The listing builds one solid part. Answer for the finished solid, in the listing's coordinates (mm). A direction names the side the tool comes from. Coordinates: 2 decimals unless noted, no trailing zeros. Write each loop counter-clockwise with the first axis right and the second up, starting at its lowest first coordinate (ties: lowest second). Pieces come first, ordered by that corner, then holes.
from build123d import *

# Parameters (mm, degrees)
SKETCH1_W           = 22.6
SKETCH1_H           = 12.33
BOSS_EXTRUDE1_DEPTH = 16.09
SKETCH2_W           = 32.3
SKETCH2_H           = 12.33
BOSS_EXTRUDE2_DEPTH = 2.41
SKETCH3_W           = 22.6
SKETCH3_H           = 12.33
BOSS_EXTRUDE3_DEPTH = 4.23
BOSS_EXTRUDE4_DEPTH = 4.31
SKETCH5_R           = 3.335
BOSS_EXTRUDE5_DEPTH = 4.52
BOSS_EXTRUDE8_DEPTH = 2.18
SKETCH8_R           = 1.3
CUT_EXTRUDE3_DEPTH  = 4
SKETCH9_R           = 1.3
CUT_EXTRUDE4_DEPTH  = 4
SKETCH10_R          = 1
CUT_EXTRUDE5_DEPTH  = 10


with BuildPart() as part:
    # Sketch1 → Boss-Extrude1 (new body)
    with BuildSketch(Plane(origin=(0, 0, 0), x_dir=(1, 0, 0), z_dir=(0, 1, 0))):
        with Locations((11.3, 6.165)):
            Rectangle(SKETCH1_W, SKETCH1_H)
    extrude(amount=BOSS_EXTRUDE1_DEPTH)

    # Sketch2 → Boss-Extrude2 (add)
    with BuildSketch(Plane(origin=(0, 16.09, 0), x_dir=(1, 0, 0), z_dir=(0, 1, 0))):
        with Locations((11.25, 6.165)):
            Rectangle(SKETCH2_W, SKETCH2_H)
    extrude(amount=BOSS_EXTRUDE2_DEPTH)

    # Sketch3 → Boss-Extrude3 (add)
    with BuildSketch(Plane(origin=(0, 18.5, 0), x_dir=(1, 0, 0), z_dir=(0, 1, 0))):
        with Locations((11.3, 6.165)):
            Rectangle(SKETCH3_W, SKETCH3_H)
    extrude(amount=BOSS_EXTRUDE3_DEPTH)

    # Sketch4 → Boss-Extrude4 (add)
    with BuildSketch(Plane(origin=(0, 22.73, 0), x_dir=(1, 0, 0), z_dir=(0, 1, 0))):
        with BuildLine():
            ThreePointArc((0, 6.165), (6.165, 12.33), (12.33, 6.165))
            ThreePointArc((12.33, 6.165), (6.165, 0), (0, 6.165))
        make_face()
    extrude(amount=BOSS_EXTRUDE4_DEPTH)

    # Sketch5 → Boss-Extrude5 (add)
    with BuildSketch(Plane(origin=(0, 27.04, 0), x_dir=(1, 0, 0), z_dir=(0, 1, 0))):
        with Locations(Location((6.165, 6.165, 0), (0, 0, 270))):
            Circle(SKETCH5_R)
    extrude(amount=BOSS_EXTRUDE5_DEPTH)

    # Sketch6 → Boss-Extrude8 (add)
    with BuildSketch(Plane(origin=(0, 31.56, 0), x_dir=(1, 0, 0), z_dir=(0, 1, 0))):
        with BuildLine():
            ThreePointArc((9.455009686, 6.710949872), (6.165, 9.5), (2.874990314, 6.710949872))
            Line((2.874990314, 6.710949872), (2.83, 6.165))
            ThreePointArc((2.83, 6.165), (6.165, 2.83), (9.5, 6.165))
            Line((9.5, 6.165), (9.455009686, 6.710949872))
        make_face()
        with BuildLine():
            ThreePointArc((8.165, 22.365), (6.165, 24.365), (4.165, 22.365))
            Line((4.165, 22.365), (2.874990314, 6.710949872))
            ThreePointArc((2.874990314, 6.710949872), (6.165, 9.5), (9.455009686, 6.710949872))
            Line((9.455009686, 6.710949872), (8.165, 22.365))
        make_face()
    extrude(amount=BOSS_EXTRUDE8_DEPTH)

    # Sketch8 → Cut-Extrude3 (cut)
    with BuildSketch(Plane(origin=(0, 18.5, 0), x_dir=(1, 0, 0), z_dir=(0, 1, 0))):
        with Locations((-3.65, 6.165)):
            Circle(SKETCH8_R)
    extrude(amount=-CUT_EXTRUDE3_DEPTH, mode=Mode.SUBTRACT)

    # Sketch9 → Cut-Extrude4 (cut)
    with BuildSketch(Plane(origin=(0, 18.5, 0), x_dir=(1, 0, 0), z_dir=(0, 1, 0))):
        with Locations((26.15, 6.165)):
            Circle(SKETCH9_R)
    extrude(amount=-CUT_EXTRUDE4_DEPTH, mode=Mode.SUBTRACT)

    # Sketch10 → Cut-Extrude5 (cut)
    with BuildSketch(Plane(origin=(0, 33.74, 0), x_dir=(1, 0, 0), z_dir=(0, 1, 0))):
        with Locations(Location((6.165, 20.865, 0), (0, 0, 270))):
            Circle(SKETCH10_R)
    extrude(amount=-CUT_EXTRUDE5_DEPTH, mode=Mode.SUBTRACT)


solid = part.part
Q1. Which of the six approach directions +Z, -Z, +X, -X, +Y, -Y give full straight-line access (tool end or side, diameter ignored) to faces 1 (the face through (-2, 18.5, -6)), 2 (the face through (0, 8, -6)), 3 (the face through (11.86, 24.85, -8.53))?
Answers below:
face 1: +Z, -Z, -X, +Y
face 2: +Z, -Z, -X, -Y
face 3: none
Q2. Determine the mould class of faces 4 (the face through (27.4, 17, -9)), 5 (the face through (6.209, 32.635, -24.365)), 6 (the face through (-2.35, 17.31, -6.11)) for opening direction Z: released by +Z, released by -Z, zero draft, split by the parting line, or undercut.
Answers below:
face 4: zero draft
face 5: released by -Z
face 6: undercut
Q3. Find the intervals of material crossed by probe 1 along Z at (x, y) = (-3.65, 16.7) (3 decimals); probe 2 along Y at (x, z) = (16.5, -7.75); probe 3 along X at (y, z) = (20, -8.5), in increasing order.
Answers below:
probe 1: z = -12.33 to -7.465, -4.865 to 0
probe 2: y = 0 to 22.73
probe 3: x = 0 to 22.6
Q4. The part is cut by section D-D, the plane x = 2. Write down the section's boundary in (y, z), then the cut area to 3 significant figures.
Answers below:
outline: (0, -12.33) - (22.73, -12.33) - (22.73, -10.71) - (27.04, -10.71) - (27.04, -1.62) - (22.73, -1.62) - (22.73, 0) - (0, 0) - close
area: 319 mm2
Q5. Given pin 1 (1.5 mm diameter, centred on x = 3, z = -15, fed in from -Y); pin 2 (4 mm diameter, centred on x = -3, z = -6, fed in from +Y); pin 3 (12 mm diameter, centred on x = 8, y = 22, fed in from -Z), each flat-ended and moving along its own axis, determine where each tip first touches the part or whether it passes through.
Answers below:
pin 1: stops at y = 31.56
pin 2: stops at y = 18.5
pin 3: stops at z = -12.33
Q6. The part is cut by section A-A, the plane x = -3.65. Write down the section's boundary in (y, z) (3 decimals), then the cut area to 3 significant figures.
Answers below:
outline: (16.09, -12.33) - (18.5, -12.33) - (18.5, -7.465) - (16.09, -7.465) - close; (16.09, -4.865) - (18.5, -4.865) - (18.5, 0) - (16.09, 0) - close
area: 23.4 mm2
Q7. The part is cut by section B-B, the plane z = -8. Write down the section's boundary in (x, y), then the cut area to 3 significant figures.
Answers below:
outline: (-4.9, 16.09) - (0, 16.09) - (0, 0) - (22.6, 0) - (22.6, 16.09) - (27.4, 16.09) - (27.4, 18.5) - (22.6, 18.5) - (22.6, 22.73) - (12.05, 22.73) - (12.05, 27.04) - (8.95, 27.04) - (8.95, 31.56) - (9.35, 31.56) - (9.35, 33.74) - (2.98, 33.74) - (2.98, 31.56) - (3.38, 31.56) - (3.38, 27.04) - (0.28, 27.04) - (0.28, 22.73) - (0, 22.73) - (0, 18.5) - (-4.9, 18.5) - close
area: 627 mm2
Q8. The part is cut by section C-C, the plane y = 21.5. Write down the section's boundary in (x, z), then the cut area to 3 significant figures.
Answers below:
outline: (0, -12.33) - (22.6, -12.33) - (22.6, 0) - (0, 0) - close
area: 279 mm2
